Read the model definition and answer for the solid it produces. Units are mm, in the model's axes. Face numbers are marked on the shaded views. A direction names the side the tool comes from. Coordinates: 2 decimals unless noted, no trailing zeros. Write each loop counter-clockwise with the first axis right and the second up, starting at its lowest first coordinate (ties: lowest second). Pieces come first, ordered by that corner, then holes. Notation, with made-up numbers: M 70.25,39.25 L 126.25,39.25 A25 cw 126.25,58.25 Z; hole C 82,-33.5 d7. An arc over 180 degrees is marked long. Write item = value, one per line.
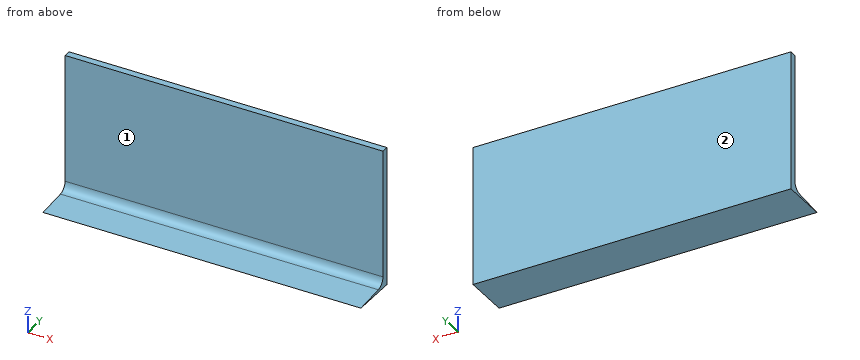
from build123d import *

# Parameters (mm, degrees)
F0_W     = 91.34856
F0_H     = 40
F1_DEPTH = 13
F3_DEPTH = 127
F4_R     = 2.54


with BuildPart() as f1:
    # F0 (on Front) → F1 (new body)
    with BuildSketch(Plane.XZ):
        with Locations((45.67428, 20)):
            Rectangle(F0_W, F0_H)
    extrude(amount=F1_DEPTH)

    # F2 (on face) → F3 (cut)
    with BuildSketch(Plane.YZ.offset(91.34856)):
        Polygon((-13, 40), (-13, 0), (-2, 0.962375), (-2, 40), align=None)
    extrude(amount=-F3_DEPTH, mode=Mode.SUBTRACT)

    # F4
    f4_edges = [f1.edges().sort_by_distance(p)[0] for p in [
        (45.67428, -2, 0.962375),
    ]]
    fillet(f4_edges, radius=F4_R)


solid = f1.part
Item 1: Find section A-A (x = 11.5). Determine the outline of the cut face in (y, z), and give its area (3 significant figures).
Worked answers:
outline = M -13,0 L 0,0 L 0,40 L -2,40 L -2,3.29 A2.54 cw -4.32,0.76 Z
area = 86.4 mm²
Item 2: Consider line 1 along Y through (x, z) = (39, 26); line 2 along Z through (x, y) = (51, -8); line 3 along Z through (x, y) = (48.5, -11). Determine where each line is inside the solid, lowest interval first. Write a range as from..to.
Worked answers:
line_1 = -2..0
line_2 = 0..0.44
line_3 = 0..0.17
Item 3: Find section B-B (z = 27). Determine the outline of the cut face in (x, y).
Worked answers:
outline = M 0,-2 L 91.35,-2 L 91.35,0 L 0,0 Z
Item 4: Which of the six approach directions +Z, -Z, +X, -X, +Y, -Y give full straight-line access (tool end or side, diameter ignored) to the marked faces 1 and 2?
Worked answers:
face_1 = +Z, +X, -X, -Y
face_2 = +Z, -Z, +X, -X, +Y
Item 5: Find section C-C (y = -8.25). Determine the outline of the cut face in (x, z).
Worked answers:
outline = M 0,0 L 91.35,0 L 91.35,0.42 L 0,0.42 Z
Item 6: Flat-ended cylindrical pins translate along their axes: pin 1 (11 mm diameter, centred on x = 36.5, z = 22, fed in from -Y); pin 2 (6 mm diameter, centred on x = 30, y = -11.5, fed in from +Z). Find the tip coordinate at first contact, or state that the pin passes through.
Worked answers:
pin_1 = -2
pin_2 = 0.39
